from build123d import *

# Parameters (mm, degrees)
BOSS_EXTRUDE2_DEPTH = 20
CUT_EXTRUDE1_DEPTH  = 21
CUT_EXTRUDE2_DEPTH  = 21


with BuildPart() as part:
    # Sketch1 → Boss-Extrude2 (new body)
    with BuildSketch(Plane(origin=(0, 0, 0), x_dir=(1, 0, 0), z_dir=(0, 1, 0))):
        Polygon((21, -13.279056191), (21, -19.052558883), (23, -19.052558883), (23, -13.279056191), (33, -7.505553499), (43, -13.279056191), (43, -19.052558883), (45, -19.052558883), (45, -13.279056191), (55, -7.505553499), (65, -13.279056191), (65, -19.052558883), (67, -19.052558883), (67, -13.279056191), (77, -7.505553499), (77, 7.400435733), (67, 13.173938425), (67, 24.720943809), (77, 30.494446501), (77, 38), (76, 38), (76, 32.226497308), (66, 26.452994616), (56, 32.226497308), (56, 38), (54, 38), (54, 32.226497308), (44, 26.452994616), (34, 32.226497308), (34, 38), (32, 38), (32, 32.226497308), (22, 26.452994616), (12, 32.226497308), (12, 38), (11, 38), (11, 30.494446501), (21, 24.720943809), (21, 13.173938425), (11, 7.400435733), (11, -7.505553499), align=None)
        Polygon((12, 5.773502692), (22, 11.547005384), (32, 5.773502692), (32, -5.773502692), (22, -11.547005384), (12, -5.773502692), align=None, mode=Mode.SUBTRACT)
        Polygon((34, 5.773502692), (44, 11.547005384), (54, 5.773502692), (54, -5.773502692), (44, -11.547005384), (34, -5.773502692), align=None, mode=Mode.SUBTRACT)
        Polygon((56, 5.773502692), (66, 11.547005384), (76, 5.773502692), (76, -5.773502692), (66, -11.547005384), (56, -5.773502692), align=None, mode=Mode.SUBTRACT)
        Polygon((43, 13.173938425), (33, 7.400435733), (23, 13.173938425), (23, 24.720943809), (33, 30.494446501), (43, 24.720943809), align=None, mode=Mode.SUBTRACT)
        Polygon((65, 13.173938425), (55, 7.400435733), (45, 13.173938425), (45, 24.720943809), (55, 30.494446501), (65, 24.720943809), align=None, mode=Mode.SUBTRACT)
    extrude(amount=BOSS_EXTRUDE2_DEPTH)

    # Sketch2 → Cut-Extrude1 (cut, through all)
    with BuildSketch(Plane(origin=(0, 20, 0), x_dir=(1, 0, 0), z_dir=(0, 1, 0))):
        Polygon((11, 6.245735195), (22, 12.596588156), (22, 25.298294078), (11, 31.649147039), (2.295872016, -19.052558883), (22, -19.052558883), (22, -12.701705922), (11, -6.350852961), align=None)
        Polygon((77, 31.649147039), (85.704127984, -19.052558883), (66, -19.052558883), (66, -12.701705922), (77, -6.350852961), (77, 6.245735195), (66, 12.596588156), (66, 25.298294078), align=None)
    extrude(amount=-CUT_EXTRUDE1_DEPTH, mode=Mode.SUBTRACT)

    # Sketch4 → Cut-Extrude2 (cut, through all)
    with BuildSketch(Plane(origin=(0, 20, 0), x_dir=(1, 0, 0), z_dir=(0, 1, 0))):
        Polygon((22, 25.298294078), (33, 31.649147039), (44, 25.298294078), (55, 31.649147039), (66, 25.298294078), (77, 31.649147039), (77, 38), (11, 38), (11, 31.649147039), align=None)
    extrude(amount=-CUT_EXTRUDE2_DEPTH, mode=Mode.SUBTRACT)


solid = part.part
Work out the finished part from the listing and answer in its coordinate system (mm). A direction names the side the tool comes from. Coordinates: 2 decimals unless noted, no trailing zeros. Write each loop counter-clockwise with the first axis right and the second up, starting at its lowest first coordinate (ties: lowest second). Pieces come first, ordered by that corner, then holes.
1. The part is cut by section B-B, the plane z = 1.5. Write down the section's boundary in (x, y).
Results list:
outline: (11, 0) - (12, 0) - (12, 20) - (11, 20) - close; (32, 0) - (34, 0) - (34, 20) - (32, 20) - close; (54, 0) - (56, 0) - (56, 20) - (54, 20) - close; (76, 0) - (77, 0) - (77, 20) - (76, 20) - close
2. For a pull along Z with two mould halves and no side action, classify faces 6 (the flat face through (65, 10, 16)), 7 (the flat face through (56, 10, 0)), 8 (the flat face through (16.577, 10.14, 9.571)) as +Z half, -Z half, draft (parallel to the pull), parting line (faces both ways), or undercut.
Results list:
face 6: draft
face 7: undercut
face 8: +Z half
3. The part is cut by section A-A, the plane z = 14. Write down the section's boundary in (x, y).
Results list:
outline: (22, 0) - (23, 0) - (23, 20) - (22, 20) - close; (43, 0) - (45, 0) - (45, 20) - (43, 20) - close; (65, 0) - (66, 0) - (66, 20) - (65, 20) - close
4. The part is cut by section D-D, the plane x = 71.5. Write down the section's boundary in (y, z).
Results list:
outline: (0, -9.42) - (20, -9.42) - (20, -8.37) - (0, -8.37) - close; (0, 8.37) - (20, 8.37) - (20, 9.53) - (0, 9.53) - close
5. Consider line 1 along X through (y, z) = (6, 1.5); line 2 along X through (y, z) = (18.25, -18); line 3 along X through (y, z) = (6, -26). Determine where each line is inside the solid, lowest interval first.
Results list:
line 1: x = 11 to 12, 32 to 34, 54 to 56, 76 to 77
line 2: x = 22 to 23, 43 to 45, 65 to 66
line 3: x = 23.22 to 25.22, 40.78 to 42.78, 45.22 to 47.22, 62.78 to 64.78
6. Flat-ended cylindrical pins translate along their axes: pin 1 (3 mm diameter, centred on y = 11, z = -13, fed in from +X); pin 2 (5 mm diameter, centred on y = 14.5, z = -10, fed in from +X); pin 3 (1 mm diameter, centred on x = 31.5, y = 3.5, fed in from +Z). Find the tip coordinate at first contact, or state that the pin passes through.
Results list:
pin 1: stops at x = 67.9
pin 2: stops at x = 74.83
pin 3: stops at z = 8.66
7. For faces 1 (the flat face through (38.42, 10.14, -28.52)), 2 (the flat face through (45, 10, 16)), 3 (the flat face through (37.93, 9.86, -27.65)), 4 (the flat face through (66, 10, -19)), 5 (the flat face through (71.423, 10.14, 9.571)), determine the directions among +Z, -Z, +X, -X, +Y, -Y from which every point of the face is accessible in a straight line to the end or side of a thin tool.
Results list:
face 1: -Z, +Y, -Y
face 2: +Z, +Y, -Y
face 3: +Y, -Y
face 4: -Z, +X, +Y, -Y
face 5: +Z, +X, +Y, -Y
8. The part is cut by section C-C, the plane x = 24.5. Write down the section's boundary in (y, z), and give its area (3 significant figures).
Results list:
outline: (0, -26.74) - (20, -26.74) - (20, -25.59) - (0, -25.59) - close; (0, -12.31) - (20, -12.31) - (20, -10.1) - (0, -10.1) - close; (0, 10.1) - (20, 10.1) - (20, 12.41) - (0, 12.41) - close
area: 113 mm2
